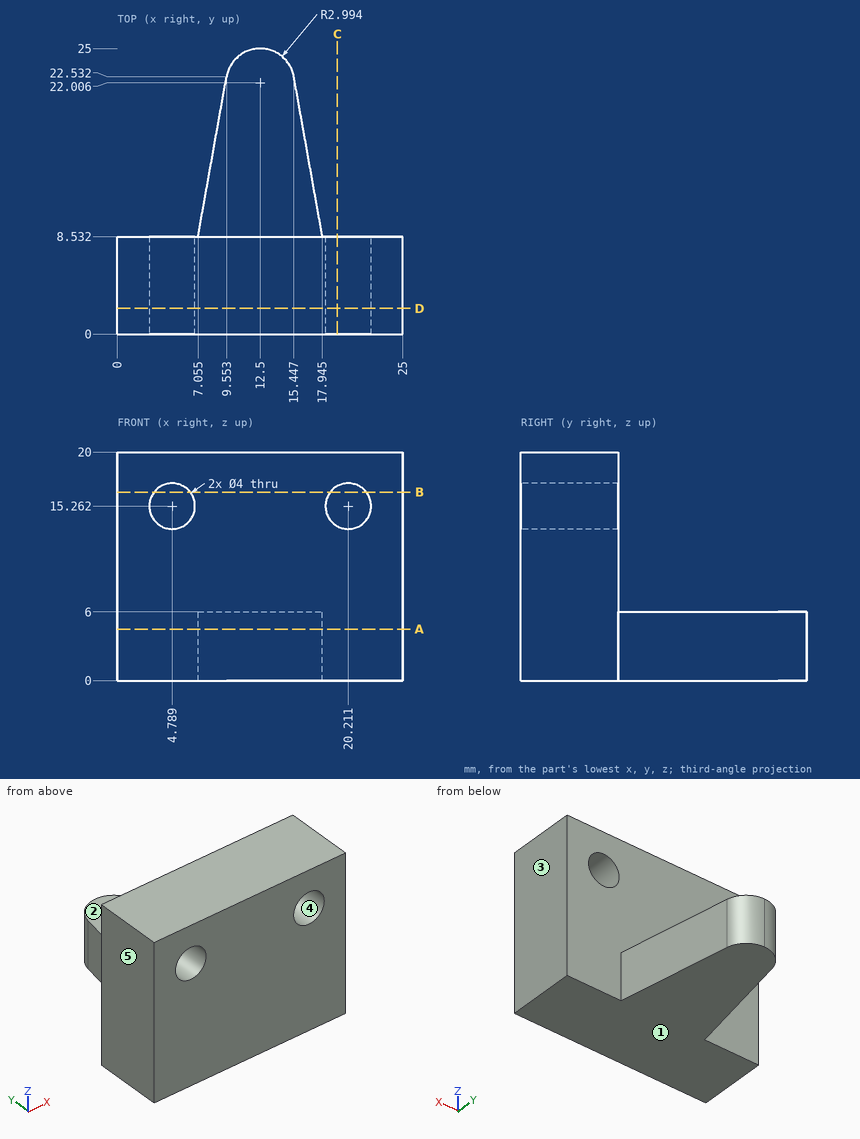
Could you check a few things on this drawing? It's one solid part, dimensions in mm from its lowest x, y, z. A direction names the side the tool comes from. Coordinates: 2 decimals unless noted, no trailing zeros. Order: outer loops, then holes, each group sorted by start corner. A loop starts at its lowest first (then second) coordinate and runs counter-clockwise, first axis right, second up.
1) We'd pull the mould along X, two halves only. Please class the marked faces 3, 4 and 5: +X half, -X half, draft (parallel to the pull), parting line (faces both ways), or undercut.
2) Which directions (+Z, -Z, +X, -X, +Y, -Y) give clear straight access to the entire face, cutting with the end or side of a thin tool? Please do the marked faces 1 and 2.
3) Imagine slicing it at B-B on z = 16.5. List the corners of the cut face in (x, y) for me, and give its area (3 significant figures).
4) Imagine slicing it at C-C on x = 19.25. List the corners of the cut face in (y, z) for me (1 decimal).
5) I need wall thicknesses on line 1 (Y direction, x = 2.75, z = 4); line 2 (Z direction, x = 8, y = 12.75); line 3 (X direction, y = 8.5, z = 16). Which ranges of each line are inside material? Lowest first, please.
6) Will these pins go through, and if not, where does the flat tip stop? pin 1 (8 mm diameter, centred on y = 15, z = 15, fed in from -X); pin 2 (4 mm diameter, centred on x = 8, z = 2, fed in from +Y) (1 decimal); pin 3 (5 mm diameter, centred on x = 4.79, z = 15.26, fed in from +Y); pin 4 (1.5 mm diameter, centred on y = 14.5, z = 4, fed in from -X).
7) Imagine slicing it at A-A on z = 4.5. List the corners of the cut face in (x, y) for me (1 decimal), and give its area (3 significant figures).
8) Imagine slicing it at D-D on y = 2.25. List the corners of the cut face in (x, z) for me, and give its area (3 significant figures).
Response values:
1. face 3: +X half
1. face 4: undercut
1. face 5: -X half
2. face 1: -Z, +X, -X, +Y, -Y
2. face 2: +Z, +X, -X, +Y
3. outline: (0, 0) - (3.22, 0) - (3.22, 8.53) - (0, 8.53) - close; (6.36, 0) - (18.64, 0) - (18.64, 8.53) - (6.36, 8.53) - close; (21.78, 0) - (25, 0) - (25, 8.53) - (21.78, 8.53) - close
3. area: 160 mm2
4. outline: (0, 0) - (8.5, 0) - (8.5, 13.5) - (0, 13.5) - close; (0, 17) - (8.5, 17) - (8.5, 20) - (0, 20) - close
5. line 1: y = 0 to 8.53
5. line 2: z = 0 to 6
5. line 3: x = 0 to 2.93, 6.65 to 18.35, 22.07 to 25
6. pin 1: passes through
6. pin 2: stops at y = 23.7
6. pin 3: stops at y = 8.53
6. pin 4: stops at x = 7.99
7. outline: (0, 0) - (25, 0) - (25, 8.5) - (17.9, 8.5) - (15.4, 22.5) arc R3 ccw to (12.5, 25) arc R3 ccw to (9.6, 22.5) - (7.1, 8.5) - (0, 8.5) - close
7. area: 342 mm2
8. outline: (0, 0) - (25, 0) - (25, 20) - (0, 20) - close; hole circle Ø4 at (4.79, 15.26); hole circle Ø4 at (20.21, 15.26)
8. area: 475 mm2
